Here's how the part is built. I have some questions about the finished solid (model axes, mm). Give positions to 0.01 mm unless a question says otherwise; leave off trailing zeros. Loops run counter-clockwise (first coordinate to the right, second up) from the corner with the lowest first, then second, coordinate; pieces in that order, holes last. Notation, with made-up numbers: (72, 4.5) -> (106, 4.5) arc R16 ccw to (106, 24.5) -> close; hole circle Ø8 at (72.5, 65.25). An arc over 180 degrees is marked (long way). Answer in a Markdown table with one row per item. Add a question column.
Item 1: If we section it at B-B (z = 0.9): Write out the boundary of the cut face in (x, y).
Item 2: For P1, Ø1, axis at x = 5.5, z = 0.5, coming from the -Y side; P2, Ø3, axis at x = -21, z = 3.5, coming from the -Y side; P3, Ø2, axis at x = -18, z = 0.5, coming from the -Y side, each with a flat end and sliding along its axis, tell me the tip position at first contact or that it passes through.
Item 3: We'd pull the mould along X, two halves only. Please class faces 1 (the face through (-8.67, -39.05, 2.46)), 2 (the face through (-37.65, 0.07, 2.46)), 3 (the face through (34.35, 0.07, 2.46)), 4 (the face through (17, -17, 5)): released by +X, released by -X, zero draft, split by the parting line, or undercut.
Item 4: If I drill on line 1 (Y direction, x = 0, z = 1.7); line 2 (Y direction, x = 1.5, z = 0.7); line 3 (Y direction, x = 15, z = 4), over which ranges is the centre line in solid material (lowest first)?
Item 5: If we section it at D-D (y = -15.5): Write out the boundary of the cut face in (x, z).
Item 6: If we section it at C-C (x = 0.5): Write out the boundary of the cut face in (y, z), then the cut area to 3 significant figures.
Item 7: If we section it at A-A (y = 0): Write out the boundary of the cut face in (x, z).
```python
from build123d import *

# Parameters (mm, degrees)
ESKIZ_KONTUR_R        = 40
PLASTINA_DEPTH        = 5
OTVERSTIYA_DEPTH      = 57.789083458
OTVERSTIYA_DEPTH_BACK = 57.789083458
ESKIZ_OTVERSTIYA_R    = 1.65
ESKIZ_OTVERSTIYA_R_2  = 23.75


with BuildPart() as part:
    # Eskiz_kontur → Plastina (new body)
    with BuildSketch(Plane.XY):
        Circle(ESKIZ_KONTUR_R)
    extrude(amount=PLASTINA_DEPTH)

    # Eskiz_otverstiya → Otverstiya (cut, two sides: drawn at the far end of the back side and taken through both)
    with BuildSketch(Plane.XY.offset(-OTVERSTIYA_DEPTH_BACK)):
        with Locations((0, -36)):
            Circle(ESKIZ_OTVERSTIYA_R)
        Circle(ESKIZ_OTVERSTIYA_R_2)
        with Locations((-36, 0)):
            Circle(ESKIZ_OTVERSTIYA_R)
        with Locations((36, 0)):
            Circle(ESKIZ_OTVERSTIYA_R)
        with Locations((0, 36)):
            Circle(ESKIZ_OTVERSTIYA_R)
    extrude(amount=OTVERSTIYA_DEPTH + OTVERSTIYA_DEPTH_BACK, mode=Mode.SUBTRACT)


solid = part.part
```
Recorded:
| question | item | result |
|---|---|---|
| 1 | outline | circle Ø80 at (0, 0); hole circle Ø3.3 at (-36, 0); hole circle Ø47.5 at (0, 0); hole circle Ø3.3 at (0, -36); hole circle Ø3.3 at (0, 36); hole circle Ø3.3 at (36, 0) |
| 2 | P1 | stops at y = -39.69 |
| 2 | P2 | stops at y = -34.92 |
| 2 | P3 | stops at y = -36.21 |
| 3 | face 1 | split by the parting line |
| 3 | face 2 | undercut |
| 3 | face 3 | undercut |
| 3 | face 4 | zero draft |
| 4 | line 1 | y = -40 to -37.65, -34.35 to -23.75, 23.75 to 34.35, 37.65 to 40 |
| 4 | line 2 | y = -39.97 to -36.69, -35.31 to -23.7, 23.7 to 35.31, 36.69 to 39.97 |
| 4 | line 3 | y = -37.08 to -18.41, 18.41 to 37.08 |
| 5 | outline | (-36.87, 0) -> (-17.99, 0) -> (-17.99, 5) -> (-36.87, 5) -> close; (17.99, 0) -> (36.87, 0) -> (36.87, 5) -> (17.99, 5) -> close |
| 6 | outline | (-40, 0) -> (-37.57, 0) -> (-37.57, 5) -> (-40, 5) -> close; (-34.43, 0) -> (-23.74, 0) -> (-23.74, 5) -> (-34.43, 5) -> close; (23.74, 0) -> (34.43, 0) -> (34.43, 5) -> (23.74, 5) -> close; (37.57, 0) -> (40, 0) -> (40, 5) -> (37.57, 5) -> close |
| 6 | area | 131 mm^2 |
| 7 | outline | (-40, 0) -> (-37.65, 0) -> (-37.65, 5) -> (-40, 5) -> close; (-34.35, 0) -> (-23.75, 0) -> (-23.75, 5) -> (-34.35, 5) -> close; (23.75, 0) -> (34.35, 0) -> (34.35, 5) -> (23.75, 5) -> close; (37.65, 0) -> (40, 0) -> (40, 5) -> (37.65, 5) -> close |
